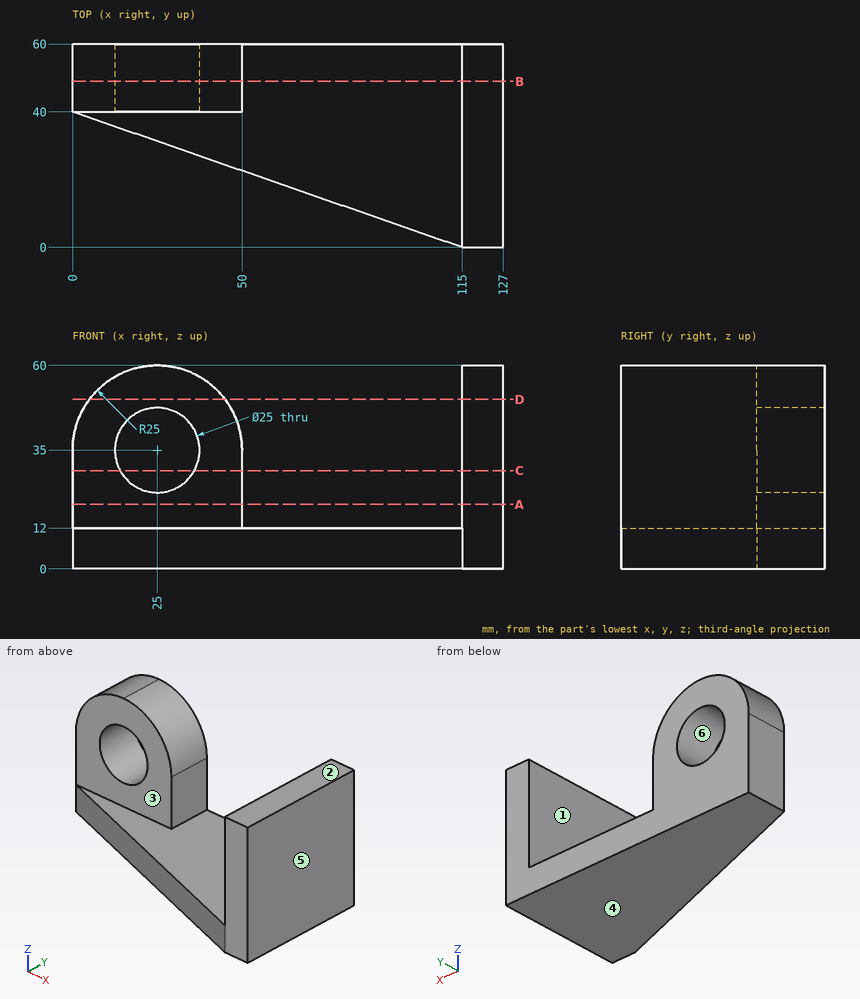
Design review of the part shown in the three views and the two pictorial views. Dimensions are in mm from the part's minimum x, y and z. A direction names the side the tool comes from. Coordinates: 2 decimals unless noted, no trailing zeros. Loops run counter-clockwise (first coordinate to the right, second up) from the corner with the lowest first, then second, coordinate; pieces in that order, holes last.
(1) Insertion check: P1, Ø1.5, axis at x = 46, y = 47, coming from the +Z side; P2, Ø1, axis at y = 8.5, z = 19, coming from the -X side; P3, Ø24, axis at x = 22.5, z = 25, coming from the -Y side. Each pin has a flat end and moves straight along its axis. Give the tip position at first contact, or say it passes through.
Determined:
P1: stops at z = 49.66
P2: stops at x = 115
P3: stops at y = 40
(2) Tool access review of the marked faces 1, 2 and 3: name each direction out of +Z, -Z, +X, -X, +Y, -Y from which nothing blocks a thin tool from reaching the whole face with its end or side.
Determined:
face 1: +Z, +Y, -Y
face 2: +Z, +X, -X, +Y, -Y
face 3: +Z, -X, -Y
(3) Consider section A-A, the plane z = 19. Give the boundary of the cut face in (x, y), plus the area to 3 significant figures.
Determined:
outline: (0, 40) - (50, 40) - (50, 60) - (0, 60) - close; (115, 0) - (127, 0) - (127, 60) - (115, 60) - close
area: 1,720 mm2
(4) Wall thickness on L1, parallel to Y at x = 15.5, z = 21.5; L2, parallel to X at y = 15, z = 22.5; L3, parallel to Z at x = 67, y = 54: over which ranges is each line inside the solid? List them lowest first.
Determined:
L1: y = 40 to 60
L2: x = 115 to 127
L3: z = 0 to 12
(5) Consider section D-D, the plane z = 50. Give the boundary of the cut face in (x, y), plus the area to 3 significant figures.
Determined:
outline: (5, 40) - (45, 40) - (45, 60) - (5, 60) - close; (115, 0) - (127, 0) - (127, 60) - (115, 60) - close
area: 1,520 mm2
(6) Draft analysis for pull direction X (two halves, no side actions). For the marked faces 4, 5 and 6, state which applies: +X half, -X half, draft (parallel to the pull), parting line (faces both ways), or undercut.
Determined:
face 4: draft
face 5: +X half
face 6: undercut
(7) Consider section C-C, the plane z = 29. Give the boundary of the cut face in (x, y), plus the area to 3 significant figures.
Determined:
outline: (0, 40) - (14.03, 40) - (14.03, 60) - (0, 60) - close; (35.97, 40) - (50, 40) - (50, 60) - (35.97, 60) - close; (115, 0) - (127, 0) - (127, 60) - (115, 60) - close
area: 1,280 mm2
(8) Consider section B-B, the plane y = 49. Give the boundary of the cut face in (x, z).
Determined:
outline: (0, 0) - (127, 0) - (127, 60) - (115, 60) - (115, 12) - (50, 12) - (50, 35) arc R25 ccw to (25, 60) arc R25 ccw to (0, 35) - close; hole circle Ø25 at (25, 35)
